```python
from build123d import *

# Parameters (mm, degrees)
SKETCH1_R           = 1.5
SKETCH1_R_2         = 0.5
BOSS_EXTRUDE1_DEPTH = 1.5
SKETCH2_R           = 3.5
SKETCH2_R_2         = 1.5
BOSS_EXTRUDE2_DEPTH = 0.1
SKETCH3_R           = 2.75
CUT_EXTRUDE1_DEPTH  = 0.05
SKETCH4_R           = 2.75
CUT_EXTRUDE2_DEPTH  = 0.05
SKETCH5_R           = 2.75
SKETCH5_R_2         = 1.5
BOSS_EXTRUDE3_DEPTH = 1.5
FILLET1_R           = 0.5
SKETCH6_W           = 2.5
SKETCH6_H           = 3
SKETCH6_R           = 0.5
BOSS_EXTRUDE4_DEPTH = 0.1
SKETCH7_W           = 2.5
SKETCH7_H           = 3
SKETCH7_R           = 0.5
BOSS_EXTRUDE5_DEPTH = 0.1


with BuildPart() as part:
    # Sketch1 → Boss-Extrude1 (new body)
    with BuildSketch(Plane(origin=(0, 0, 0), x_dir=(1, 0, 0), z_dir=(0, 1, 0))):
        with BuildLine():
            Line((-3.75, -7.75), (-3.75, -3.307189139))
            ThreePointArc((-3.75, -3.307189139), (-5, 0), (-3.75, 3.307189139))
            Line((-3.75, 3.307189139), (-3.75, 11.807189139))
            Line((-3.75, 11.807189139), (-3.25, 12.807189139))
            Line((-3.25, 12.807189139), (-2.75, 15.807189139))
            Line((-2.75, 15.807189139), (2.75, 15.807189139))
            Line((2.75, 15.807189139), (3.25, 12.807189139))
            Line((3.25, 12.807189139), (3.75, 11.807189139))
            Line((3.75, 11.807189139), (3.75, 3.307189139))
            ThreePointArc((3.75, 3.307189139), (5, 0), (3.75, -3.307189139))
            Line((3.75, -3.307189139), (3.75, -7.75))
            ThreePointArc((3.75, -7.75), (0, -11.5), (-3.75, -7.75))
        make_face()
        with Locations((0, -7.75)):
            Circle(SKETCH1_R, mode=Mode.SUBTRACT)
        with Locations((0, 7.75)):
            Circle(SKETCH1_R, mode=Mode.SUBTRACT)
        with Locations((-1.5, 14.307189139)):
            Circle(SKETCH1_R_2, mode=Mode.SUBTRACT)
        with Locations((1.5, 14.307189139)):
            Circle(SKETCH1_R_2, mode=Mode.SUBTRACT)
        Circle(SKETCH1_R, mode=Mode.SUBTRACT)
    extrude(amount=BOSS_EXTRUDE1_DEPTH)

    # Sketch2 → Boss-Extrude2 (add)
    with BuildSketch(Plane(origin=(0, 1.5, 0), x_dir=(1, 0, 0), z_dir=(0, 1, 0))):
        Circle(SKETCH2_R)
        Circle(SKETCH2_R_2, mode=Mode.SUBTRACT)
    extrude(amount=BOSS_EXTRUDE2_DEPTH)

    # Sketch3 → Cut-Extrude1 (cut)
    with BuildSketch(Plane(origin=(0, 1.5, 0), x_dir=(1, 0, 0), z_dir=(0, 1, 0))):
        with Locations((0, -7.75)):
            Circle(SKETCH3_R)
        with Locations((0, 7.75)):
            Circle(SKETCH3_R)
    extrude(amount=-CUT_EXTRUDE1_DEPTH, mode=Mode.SUBTRACT)

    # Sketch4 → Cut-Extrude2 (cut)
    with BuildSketch(Plane.XZ):
        with Locations((0, -7.75)):
            Circle(SKETCH4_R)
        with Locations((0, 7.75)):
            Circle(SKETCH4_R)
    extrude(amount=-CUT_EXTRUDE2_DEPTH, mode=Mode.SUBTRACT)

    # Sketch5 → Boss-Extrude3 (add)
    with BuildSketch(Plane.XZ):
        Circle(SKETCH5_R)
        Circle(SKETCH5_R_2, mode=Mode.SUBTRACT)
    extrude(amount=BOSS_EXTRUDE3_DEPTH)

    # Fillet1
    fillet1_edges = [part.edges().sort_by_distance(p)[0] for p in [
        (-2.75, 0, 0),
    ]]
    fillet(fillet1_edges, radius=FILLET1_R)

    # Sketch6 → Boss-Extrude4 (add)
    with BuildSketch(Plane(origin=(0, 1.5, 0), x_dir=(1, 0, 0), z_dir=(0, 1, 0))):
        with Locations((-1.5, 14.307189139)):
            Rectangle(SKETCH6_W, SKETCH6_H)
        with Locations((-1.5, 14.307189139)):
            Circle(SKETCH6_R, mode=Mode.SUBTRACT)
        with Locations((1.5, 14.307189139)):
            Rectangle(SKETCH6_W, SKETCH6_H)
        with Locations((1.5, 14.307189139)):
            Circle(SKETCH6_R, mode=Mode.SUBTRACT)
    extrude(amount=BOSS_EXTRUDE4_DEPTH)

    # Sketch7 → Boss-Extrude5 (add)
    with BuildSketch(Plane.XZ):
        with Locations((-1.5, -14.307189139)):
            Rectangle(SKETCH7_W, SKETCH7_H)
        with Locations((-1.5, -14.307189139)):
            Circle(SKETCH7_R, mode=Mode.SUBTRACT)
        with Locations((1.5, -14.307189139)):
            Rectangle(SKETCH7_W, SKETCH7_H)
        with Locations((1.5, -14.307189139)):
            Circle(SKETCH7_R, mode=Mode.SUBTRACT)
    extrude(amount=BOSS_EXTRUDE5_DEPTH)


solid = part.part
```
Work out the finished part from the listing and answer in its coordinate system (mm). A direction names the side the tool comes from. Coordinates: 2 decimals unless noted, no trailing zeros. Write each loop counter-clockwise with the first axis right and the second up, starting at its lowest first coordinate (ties: lowest second). Pieces come first, ordered by that corner, then holes.
Q1. Determine the mould class of faces 5 (the face through (0.1, 0.7, 11.5)), 6 (the face through (0, 1, -15.807)), 7 (the face through (3.75, 1, 5)), 8 (the face through (1.2, 0.05, -8.9)) for opening direction Z: released by +Z, released by -Z, zero draft, split by the parting line, or undercut.
Q2. Each of these flat-tipped pins is pushed along its axis until it touches: pin 1 Ø3 at (x, z) = (-0.5, -11.5) entering from -Y; pin 2 Ø5 at (x, z) = (0, 7.75) entering from -Y; pin 3 Ø6 at (x, z) = (0.5, -8.5) entering from -Y. Where does it stop, or does it pass through?
Q3. A cutting plane is placed at D-D, the plane x = 0. State how many separate pieces and enclosed holes the cut face has, then the cut area to 3 significant figures.
Q4. A cutting plane is placed at A-A, the plane z = 0. Give the vertices of the cut face in (x, y), then the cut area to 3 significant figures.
Q5. Find the intervals of material crossed by line 1 (Z direction, x = 0, y = 0.5); line 2 (Z direction, x = 0, y = 1.55); line 3 (Y direction, x = -3.5, z = -9.25), in increasing order.
Q6. A cutting plane is placed at C-C, the plane y = -0.75. Give the vertices of the cut face in (x, z), then the cut area to 3 significant figures.
Q7. Which of the six approach directions +Z, -Z, +X, -X, +Y, -Y give full straight-line access (tool end or side, diameter ignored) to faces 1 (the face through (1.2, 1.45, -6.6)), 2 (the face through (-3, 0, -2)), 3 (the face through (-3.75, 1, 6)), 4 (the face through (-3.75, 1, -7))?
Q8. A cutting plane is placed at B-B, the plane y = 1.2. Give the vertices of the cut face in (x, z), then the cut area to 3 significant figures.
Findings below:
1. face 5: released by +Z
1. face 6: released by -Z
1. face 7: zero draft
1. face 8: undercut
2. pin 1: stops at y = -0.1
2. pin 2: stops at y = 0.05
2. pin 3: stops at y = 0
3. separate pieces: 4
3. enclosed holes: 0
3. area: 31.2 mm2
4. outline: (-5, 0) - (-3.25, 0) arc R0.5 cw to (-2.75, -0.5) - (-2.75, -1.5) - (-1.5, -1.5) - (-1.5, 1.6) - (-3.5, 1.6) - (-3.5, 1.5) - (-5, 1.5) - close; (1.5, -1.5) - (2.75, -1.5) - (2.75, -0.5) arc R0.5 cw to (3.25, 0) - (5, 0) - (5, 1.5) - (3.5, 1.5) - (3.5, 1.6) - (1.5, 1.6) - close
4. area: 14.8 mm2
5. line 1: z = -15.81 to -9.25, -6.25 to -1.5, 1.5 to 6.25, 9.25 to 11.5
5. line 2: z = -3.5 to -1.5, 1.5 to 3.5
5. line 3: y = 0 to 1.5
6. outline: circle Ø5.5 at (0, 0); hole circle Ø3 at (0, 0)
6. area: 16.7 mm2
7. face 1: +Y
7. face 2: -Y
7. face 3: +Z, -X, +Y, -Y
7. face 4: -Z, -X, +Y, -Y
8. outline: (-3.75, -11.81) - (-3.25, -12.81) - (-2.75, -15.81) - (2.75, -15.81) - (3.25, -12.81) - (3.75, -11.81) - (3.75, -3.31) arc R5 ccw to (3.75, 3.31) - (3.75, 7.75) arc R3.75 ccw to (-3.75, 7.75) - (-3.75, 3.31) arc R5 ccw to (-3.75, -3.31) - close; hole circle Ø1 at (-1.5, -14.31); hole circle Ø3 at (0, -7.75); hole circle Ø3 at (0, 0); hole circle Ø3 at (0, 7.75); hole circle Ø1 at (1.5, -14.31)
8. area: 182 mm2
